from build123d import *

# Parameters (mm, degrees)
F0_R      = 40
F1_DEPTH  = 20
F2_R      = 25
F3_DEPTH  = 20
F4_R      = 20
F5_DEPTH  = 20
F6_R      = 15
F7_DEPTH  = 20
F8_R      = 10.4214785956
F9_DEPTH  = 20
F10_R     = 5
F11_DEPTH = 20
F12_R     = 2.5
F13_DEPTH = 20
F14_R     = 25
F15_DEPTH = 40
F16_R     = 20
F17_DEPTH = 60


with BuildPart() as f1:
    # F0 (on Front) → F1 (new body)
    with BuildSketch(Plane.XZ):
        Circle(F0_R)
    extrude(amount=F1_DEPTH)

    # F2 (on face) → F3 (join)
    with BuildSketch(Plane(origin=(0, 0, 0), x_dir=(-1, 0, 0), z_dir=(0, 1, 0))):
        Circle(F2_R)
    extrude(amount=F3_DEPTH)

    # F4 (on face) → F5 (join)
    with BuildSketch(Plane(origin=(0, 20, 0), x_dir=(-1, 0, 0), z_dir=(0, 1, 0))):
        Circle(F4_R)
    extrude(amount=F5_DEPTH)

    # F6 (on face) → F7 (join)
    with BuildSketch(Plane(origin=(0, 40, 0), x_dir=(-1, 0, 0), z_dir=(0, 1, 0))):
        Circle(F6_R)
    extrude(amount=F7_DEPTH)

    # F8 (on face) → F9 (join)
    with BuildSketch(Plane(origin=(0, 60, 0), x_dir=(-1, 0, 0), z_dir=(0, 1, 0))):
        Circle(F8_R)
    extrude(amount=F9_DEPTH)

    # F10 (on face) → F11 (join)
    with BuildSketch(Plane(origin=(0, 80, 0), x_dir=(-1, 0, 0), z_dir=(0, 1, 0))):
        Circle(F10_R)
    extrude(amount=F11_DEPTH)

    # F12 (on face) → F13 (join)
    with BuildSketch(Plane(origin=(0, 100, 0), x_dir=(-1, 0, 0), z_dir=(0, 1, 0))):
        Circle(F12_R)
    extrude(amount=F13_DEPTH)

    # F14 (on face) → F15 (join)
    with BuildSketch(Plane.XZ.offset(20)):
        Circle(F14_R)
    extrude(amount=F15_DEPTH)

    # F16 (on face) → F17 (cut)
    with BuildSketch(Plane.XZ.offset(60)):
        Circle(F16_R)
    extrude(amount=-F17_DEPTH, mode=Mode.SUBTRACT)


solid = f1.part
Here's how the part is built. I have some questions about the finished solid (model axes, mm). A direction names the side the tool comes from. Coordinates: 2 decimals unless noted, no trailing zeros. Write each loop counter-clockwise with the first axis right and the second up, starting at its lowest first coordinate (ties: lowest second). Pieces come first, ordered by that corner, then holes.
1) Thinking about a two-plate mould opening in Z: for faces 1 (the face through (0, 120, 0)), 2 (the face through (0, 0, 0)), 3 (the face through (14.985, 49.86, 0.66)), which applies, +Z half, -Z half, draft (parallel to the pull), parting line (faces both ways), or undercut?
Filled in:
face 1: draft
face 2: undercut
face 3: parting line
2) If we section it at A-A (y = -47): List the corners of the cut face in (x, z) for me, plus the area to 3 significant figures.
Filled in:
outline: circle Ø50 at (0, 0); hole circle Ø40 at (0, 0)
area: 707 mm2
3) Which directions (+Z, -Z, +X, -X, +Y, -Y) give clear straight access to the entire face, cutting with the end or side of a thin tool? Please do faces 4 (the face through (-3.1, 60, 10.2)), 5 (the face through (23.846, -39.72, 7.509)), 6 (the face through (-11, -60, 17)).
Filled in:
face 4: +Y
face 5: -Y
face 6: +Z, -Z, +X, -X, -Y
4) I'm going to push flat-ended pins straight in: pin 1 (2 mm diameter, centred on x = -18.5, y = 6.5, fed in from -Z); pin 2 (4 mm diameter, centred on x = 4, z = -32, fed in from -Y); pin 3 (10 mm diameter, centred on x = 1.5, z = 11.5, fed in from +Y). Where does each tip first touch, or does it pass through?
Filled in:
pin 1: stops at z = -17.85
pin 2: stops at y = -20
pin 3: stops at y = 80
5) If we section it at C-C (y = 68): List the corners of the cut face in (x, z) for me, plus the area to 3 significant figures.
Filled in:
outline: circle Ø20.84 at (0, 0)
area: 341 mm2
6) If we section it at D-D (z = -8): List the corners of the cut face in (x, y) for me.
Filled in:
outline: (-39.19, -20) - (-23.69, -20) - (-23.69, -60) - (-18.33, -60) - (-18.33, 0) - (18.33, 0) - (18.33, -60) - (23.69, -60) - (23.69, -20) - (39.19, -20) - (39.19, 0) - (23.69, 0) - (23.69, 20) - (18.33, 20) - (18.33, 40) - (12.69, 40) - (12.69, 60) - (6.68, 60) - (6.68, 80) - (-6.68, 80) - (-6.68, 60) - (-12.69, 60) - (-12.69, 40) - (-18.33, 40) - (-18.33, 20) - (-23.69, 20) - (-23.69, 0) - (-39.19, 0) - close
7) If we section it at B-B (x = -23): List the corners of the cut face in (y, z) for me.
Filled in:
outline: (-60, -9.8) - (-20, -9.8) - (-20, -32.73) - (0, -32.73) - (0, -9.8) - (20, -9.8) - (20, 9.8) - (0, 9.8) - (0, 32.73) - (-20, 32.73) - (-20, 9.8) - (-60, 9.8) - close
8) If I drill on line 1 (Z direction, x = 0, y = -15); line 2 (Z direction, x = 0, y = -48); line 3 (Y direction, x = 19.5, z = 6), over which ranges is the centre line in solid material (lowest first)?
Filled in:
line 1: z = -40 to -20, 20 to 40
line 2: z = -25 to -20, 20 to 25
line 3: y = -60 to 20
